from build123d import *

# Parameters (mm, degrees)
SKETCH1_W           = 101.6
SKETCH1_H           = 31.75
BOSS_EXTRUDE1_DEPTH = 18.288
SKETCH2_W           = 22.098
SKETCH2_H           = 31.75
CUT_EXTRUDE1_DEPTH  = 14.9098
SKETCH3_W           = 36.3728
SKETCH3_H           = 11.5316
CUT_EXTRUDE2_DEPTH  = 109.004969534
SKETCH4_W           = 25.37968
SKETCH4_H           = 3.3782
BOSS_EXTRUDE2_DEPTH = 50.8
SKETCH5_R           = 6.3246
BOSS_EXTRUDE3_DEPTH = 47.498


with BuildPart() as part:
    # Sketch1 → Boss-Extrude1 (new body)
    with BuildSketch(Plane(origin=(0, 0, 0), x_dir=(1, 0, 0), z_dir=(0, 1, 0))):
        with Locations((50.8, 15.875)):
            Rectangle(SKETCH1_W, SKETCH1_H)
    extrude(amount=BOSS_EXTRUDE1_DEPTH)

    # Sketch2 → Cut-Extrude1 (cut)
    with BuildSketch(Plane(origin=(0, 18.288, 0), x_dir=(1, 0, 0), z_dir=(0, 1, 0))):
        with Locations((50.8, 15.875)):
            Rectangle(SKETCH2_W, SKETCH2_H)
    extrude(amount=-CUT_EXTRUDE1_DEPTH, mode=Mode.SUBTRACT)

    # Sketch3 → Cut-Extrude2 (cut, through all)
    with BuildSketch(Plane.XY):
        with Locations((21.5646, 9.144)):
            Rectangle(SKETCH3_W, SKETCH3_H)
        with Locations((80.0354, 9.144)):
            Rectangle(SKETCH3_W, SKETCH3_H)
    extrude(amount=-CUT_EXTRUDE2_DEPTH, mode=Mode.SUBTRACT)

    # Sketch4 → Boss-Extrude2 (add)
    with BuildSketch(Plane.XZ):
        with Locations((50.8, -15.875)):
            Rectangle(SKETCH4_W, SKETCH4_H)
    extrude(amount=BOSS_EXTRUDE2_DEPTH)

    # Sketch5 → Boss-Extrude3 (add)
    with BuildSketch(Plane.XY.offset(-14.1859)):
        with Locations(Location((50.8, -44.45, 0), (0, 0, 180))):
            Circle(SKETCH5_R)
    extrude(amount=BOSS_EXTRUDE3_DEPTH)


solid = part.part
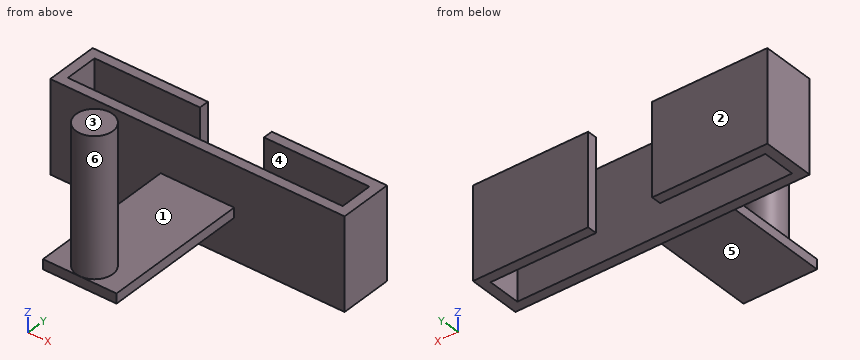
The model under review builds one solid part; all positions refer to its coordinate system, in mm. Face numbers are marked on the shaded views. A direction names the side the tool comes from. Round coordinates to 2 decimals unless told otherwise and drop trailing zeros. Order: outer loops, then holes, each group sorted by start corner. A loop starts at its lowest first (then second) coordinate and runs counter-clockwise, first axis right, second up. Notation, with made-up numbers: (52.5, 36.25) -> (90.5, 36.25) arc R27 ccw to (90.5, 54.25) -> close; hole circle Ø6 at (-26.5, 32). An arc over 180 degrees is marked (long way). Use CSV: the item, a comma, the result in double quotes. Start each with the question number.
(1) Mouldability with a two-part tool opening along Y and no side actions: class the marked faces 1, 2 and 3 as pulls with the +Y half, pulls with the -Y half, needs draft (parallel to the pull), parting line crosses it, or undercut.
(2) Consider section B-B on z = -3. Write out the cut boundary in (x, y).
(3) Insertion check: pin 1 (1.5 mm diameter, centred on x = 50.5, y = -30.5, fed in from +Z); pin 2 (12 mm diameter, centred on x = 65, y = -14, fed in from -Z); pin 3 (1.7 mm diameter, centred on y = -25, z = -15.5, fed in from -X). Each pin has a flat end and moves straight along its axis. Give the tip position at first contact, or say it passes through.
(4) Tool access review of the marked faces 4, 5 and 6: name each direction out of +Z, -Z, +X, -X, +Y, -Y from which nothing blocks a thin tool from reaching the whole face with its end or side.
(5) Consider section A-A on x = 16. Write out the cut boundary in (y, z).
(6) Consider section D-D on y = -44.45. Write out the cut boundary in (x, z), and give its area (3 significant figures).
(7) Wall thickness on probe 1 along X at (y, z) = (6.5, -18.5); probe 2 along Y at (x, z) = (19.5, -2); probe 3 along X at (y, z) = (-45, 17.5): over which ranges is each line inside the solid? List them lowest first. Write a range as from..to.
Responses:
1,face 1,"undercut"
1,face 2,"pulls with the +Y half"
1,face 3,"needs draft"
2,outline,"(0, 0) -> (101.6, 0) -> (101.6, 18.29) -> (61.85, 18.29) -> (61.85, 14.91) -> (98.22, 14.91) -> (98.22, 3.38) -> (3.38, 3.38) -> (3.38, 14.91) -> (39.75, 14.91) -> (39.75, 18.29) -> (0, 18.29) -> close; circle Ø12.65 at (50.8, -44.45)"
3,pin 1,"z = -14.19"
3,pin 2,"z = -17.56"
3,pin 3,"x = 38.11"
4,face 4,"+Z, -Z"
4,face 5,"-Z, +X, -X, -Y"
4,face 6,"+Z"
5,outline,"(0, -31.75) -> (3.38, -31.75) -> (3.38, 0) -> (0, 0) -> close; (14.91, -31.75) -> (18.29, -31.75) -> (18.29, 0) -> (14.91, 0) -> close"
6,outline,"(38.11, -17.56) -> (63.49, -17.56) -> (63.49, -14.19) -> (57.12, -14.19) -> (57.12, 33.31) -> (44.48, 33.31) -> (44.48, -14.19) -> (38.11, -14.19) -> close"
6,area,"687 mm²"
7,probe 1,"0..3.38, 98.22..101.6"
7,probe 2,"0..3.38, 14.91..18.29"
7,probe 3,"44.5..57.1"
